For this review, take the finished solid that the model builds, in its own axes (mm). Face numbers are marked on the shaded views. Give positions to 0.01 mm unless a question says otherwise; leave off trailing zeros. Order: outer loops, then holes, each group sorted by start corner. A loop starts at its lowest first (then second) coordinate and runs counter-clockwise, first axis right, second up. Notation, with made-up numbers: M -28.75,65 L -3.75,65 A18 cw -3.75,97 Z; hole C 48,58.25 d1. An arc over 180 degrees is marked long. Answer as CSV lines item,"result". Start each with the question number.
1. We need section B-B, the plane x = -15. Give the boundary of the cut face in (y, z).
2. For line 1 along Z through (x, y) = (-7.5, -6); line 2 along X through (y, z) = (5.5, -0.5); line 3 along Z through (x, y) = (-16, -2), list the stretches that pass through material, from the lowest coordinate up.
3. We need section A-A, the plane x = -8.5. Give the boundary of the cut face in (y, z), and give its area (3 significant figures).
4. Mouldability with a two-part tool opening along Y and no side actions: class the marked faces 1, 2, 3 and 4 as pulls with the +Y half, pulls with the -Y half, needs draft (parallel to the pull), parting line crosses it, or undercut.
5. Clearance check with flat-ended pins moving along their axes: P1, Ø3, axis at x = -10.5, z = 1.5, coming from the +Y side; P2, Ø2, axis at y = -7.07, z = 7.07, coming from the -X side; P3, Ø6, axis at y = 1, z = 1.5, coming from the +X side; P4, Ø16, axis at y = 0, z = 0, coming from the -X side. State where each tip first meets the part, or that it passes through.
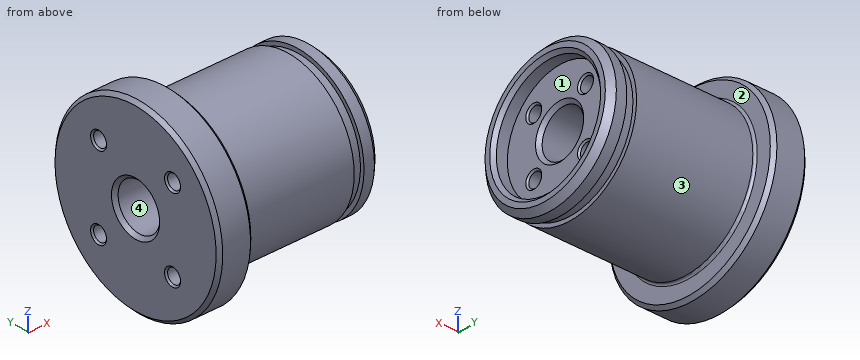
from build123d import *

# Parameters (mm, degrees)
SKETCH_2_W               = 1.7
SKETCH_2_H               = 0.7
CHAMFER_1_SIZE           = 1
FILLET_1_R               = 0.4
SKETCH_5_W               = 2.5
SKETCH_5_H               = 10
PATTERN_CIRCULAR_1_COUNT = 4
CHAMFER_2_SIZE           = 0.6
SKETCH_6_W               = 31
SKETCH_6_H               = 4
CHAMFER_3_SIZE           = 0.6
PATTERN_CIRCULAR_2_COUNT = 4
CHAMFER_4_SIZE           = 0.6


with BuildPart() as part:
    # Эскиз1 → Повернуть1 (revolve)
    with BuildSketch(Plane.XY):
        Polygon((0, 0), (0, 12.5), (-25, 12.5), (-25, 16), (-31, 16), (-31, 0), align=None)
    revolve(axis=Axis((0, 0, 0), (1, 0, 0)))

    # Эскиз2 → Вырез-Повернуть1 (revolve, cut)
    with BuildSketch(Plane.XY):
        with Locations((-3.65, 12.15)):
            Rectangle(SKETCH_2_W, SKETCH_2_H)
    revolve(axis=Axis((0, 0, 0), (-1, 0, 0)), mode=Mode.SUBTRACT)

    # Фаска1
    chamfer_1_edges = [part.edges().sort_by_distance(p)[0] for p in [
        (0, -12.5, 0),
    ]]
    chamfer(chamfer_1_edges, length=CHAMFER_1_SIZE)

    # Скругление1
    fillet_1_edges = [part.edges().sort_by_distance(p)[0] for p in [
        (-25, -12.5, 0),
    ]]
    fillet(fillet_1_edges, radius=FILLET_1_R)

    # Эскиз5 → Вырез-Повернуть2 (revolve, cut)
    with BuildSketch(Plane.XY):
        with Locations((-1.25, 5)):
            Rectangle(SKETCH_5_W, SKETCH_5_H)
    revolve(axis=Axis((0, 0, 0), (-1, 0, 0)), mode=Mode.SUBTRACT)

    # Эскиз4 → Отверстие обработанное метчиком M31 (revolve, cut)
    with BuildSketch(Plane(origin=(-2.5, 4.949747468, -4.949747468), x_dir=(0, 0, -1), z_dir=(0, 1, 0))):
        Polygon((0, 0), (0, 7.751075774), (1.25, 7), (1.25, 0.275), (1.525, 0), align=None)
    hole_wizard_m31 = revolve(axis=Axis((3.85, 4.949747468, -4.949747468), (-1, 0, 0)), mode=Mode.SUBTRACT)

    # Круговой массив1: Отверстие обработанное метчиком M31 ×4 about axis
    pattern_circular_1_axis = Axis((0, 0, 0), (1, 0, 0))
    for i in range(1, PATTERN_CIRCULAR_1_COUNT):
        add(hole_wizard_m31.rotate(pattern_circular_1_axis, i * 360 / PATTERN_CIRCULAR_1_COUNT), mode=Mode.SUBTRACT)

    # Фаска2
    chamfer_2_edges = [part.edges().sort_by_distance(p)[0] for p in [
        (0, -10, 0),
    ]]
    chamfer(chamfer_2_edges, length=CHAMFER_2_SIZE)

    # Эскиз6 → Вырез-Повернуть3 (revolve, cut)
    with BuildSketch(Plane.XY):
        with Locations((-15.5, 2)):
            Rectangle(SKETCH_6_W, SKETCH_6_H)
    revolve(axis=Axis((0, 0, 0), (-1, 0, 0)), mode=Mode.SUBTRACT)

    # Фаска3
    chamfer_3_edges = [part.edges().sort_by_distance(p)[0] for p in [
        (-31, -4, 0),
        (-2.5, -4, 0),
    ]]
    chamfer(chamfer_3_edges, length=CHAMFER_3_SIZE)

    # Эскиз8 → Отверстие обработанное метчиком M32 (revolve, cut)
    with BuildSketch(Plane(origin=(-31, 7.071067812, 7.071067812), x_dir=(0, 0, 1), z_dir=(0, 1, 0))):
        Polygon((0, 0), (0, 8.751075774), (1.25, 8), (1.25, 0.275), (1.525, 0), align=None)
    hole_wizard_m32 = revolve(axis=Axis((-37.35, 7.071067812, 7.071067812), (1, 0, 0)), mode=Mode.SUBTRACT)

    # Круговой массив2: Отверстие обработанное метчиком M32 ×4 about axis
    pattern_circular_2_axis = Axis((0, 0, 0), (1, 0, 0))
    for i in range(1, PATTERN_CIRCULAR_2_COUNT):
        add(hole_wizard_m32.rotate(pattern_circular_2_axis, i * 360 / PATTERN_CIRCULAR_2_COUNT), mode=Mode.SUBTRACT)

    # Фаска4
    chamfer_4_edges = [part.edges().sort_by_distance(p)[0] for p in [
        (-31, -16, 0),
        (-25, -16, 0),
    ]]
    chamfer(chamfer_4_edges, length=CHAMFER_4_SIZE)


solid = part.part
Result set:
1,outline,"C 0,0 d25; hole C 0,0 d8"
2,line 1,"-10.97 to -5.63, -4.27 to 4.27, 5.63 to 10.97"
2,line 2,"-31 to -2.5"
2,line 3,"-12.34 to -3.46, 3.46 to 12.34"
3,outline,"C 0,0 d25; hole C -4.95,-4.95 d2.5; hole C -4.95,4.95 d2.5; hole C 0,0 d8; hole C 4.95,-4.95 d2.5; hole C 4.95,4.95 d2.5"
3,area,"421 mm2"
4,face 1,"undercut"
4,face 2,"needs draft"
4,face 3,"parting line crosses it"
4,face 4,"undercut"
5,P1,"y = 12.5"
5,P2,"x = -22.85"
5,P3,"x = -2.5"
5,P4,"x = -31"
